Autodesk Inventor part; units mm, degrees
ref_plane "YZ Plane" through (0, 0, 0) normal (1, 0, 0) x (0, 1, 0)
ref_plane "XZ Plane" through (0, 0, 0) normal (0, 1, 0) x (-1, 0, 0)
ref_plane "XY Plane" through (0, 0, 0) normal (0, 0, 1) x (1, 0, 0)
sketch "Sketch1" plane through (0, 0, 0) normal (0, 0, 1) x (1, 0, 0)
  line L0 (0, 0) -> (128, 0)
  line L1 (128, 0) -> (128, 22.5)
  line L2 (0, 23.5) -> (0, 0)
  line L3 (68, 23.5) -> (68, 22.5)
  line L4 (68, 22.5) -> (128, 22.5)
  line L5 (33, 23.5) -> (33, 14.5)
  line L6 (33, 14.5) -> (44, 14.5)
  line L7 (44, 14.5) -> (44, 23.5)
  line L8 (68, 23.5) -> (44, 23.5)
  line L9 (33, 23.5) -> (0, 23.5)
  line L10 (72, 14.5) -> (72, 8)
  line L11 (72, 8) -> (76, 4)
  line L12 (76, 4) -> (118, 4)
  line L13 (118, 4) -> (122, 8)
  line L14 (122, 8) -> (122, 14.5)
  line L15 (122, 14.5) -> (118, 18.5)
  line L16 (118, 18.5) -> (76, 18.5)
  line L17 (76, 18.5) -> (72, 14.5)
  line L18 (68, 22.5) -> (68, 0) construction
  circle A0 centre (5.5, 19) radius 2.25
  circle A1 centre (25.5, 19) radius 2.25
  circle A2 centre (15.5, 19.599) radius 2.75
  circle A3 centre (38.5, 19.599) radius 7.5 construction
  circle A4 centre (38.5, 19.599) radius 4 construction
  point P0 (33, 19)
  dimension "d0" = 128
  dimension "d1" = 23.5
  dimension "d2" = 22.5
  dimension "d3" = 60
  dimension "d4" = 11
  dimension "d5" = 9
  dimension "d6" = 33
  dimension "d7" = 45
  dimension "d8" = 4
  dimension "d9" = 4
  dimension "d10" = 6
  dimension "d11" = 4
  dimension "d12" = 4
  dimension "d13" = 4.5
  dimension "d14" = 4.5
  dimension "d15" = 5.5
  dimension "d16" = 20
  dimension "d17" = 5.5
  dimension "d18" = 8
  dimension "d19" = 15
  dimension "d20" = 10
extrude "Extrusion1" add sketch "Sketch1" along normal blind 6.5
sketch "Sketch2" plane through (0, 0, 6.5) normal (0, 0, 1) x (1, 0, 0)
  line L0 (0, 0) -> (128, 0)
  line L1 (128, 0) -> (128, 22.5)
  line L2 (128, 22.5) -> (68, 22.5)
  line L3 (33, 23.5) -> (0, 23.5)
  line L4 (0, 23.5) -> (0, 0)
  line L5 (25, 23.5) -> (33, 23.5)
  line L6 (33, 23.5) -> (33, 29.5)
  line L7 (31, 31.5) -> (27, 31.5)
  line L8 (25, 29.5) -> (25, 23.5)
  line L9 (94, 22.5) -> (102, 22.5)
  line L10 (102, 22.5) -> (102, 27)
  line L11 (100, 29) -> (96, 29)
  line L12 (94, 27) -> (94, 22.5)
  line L13 (15, 0) -> (23, 0)
  line L14 (23, 0) -> (23, -19)
  line L15 (21, -21) -> (17, -21)
  line L16 (15, -19) -> (15, 0)
  line L17 (44, 0) -> (52, 0)
  line L18 (52, 0) -> (52, -19)
  line L19 (50, -21) -> (46, -21)
  line L20 (44, -19) -> (44, 0)
  line L21 (94, 0) -> (102, 0)
  line L22 (102, 0) -> (102, -4.5)
  line L23 (100, -6.5) -> (96, -6.5)
  line L24 (94, -4.5) -> (94, 0)
  arc A0 (27, 31.5) -> (25, 29.5) centre (27, 29.5) ccw
  arc A1 (33, 29.5) -> (31, 31.5) centre (31, 29.5) ccw
  arc A2 (96, 29) -> (94, 27) centre (96, 27) ccw
  arc A3 (102, 27) -> (100, 29) centre (100, 27) ccw
  arc A4 (15, -19) -> (17, -21) centre (17, -19) ccw
  arc A5 (21, -21) -> (23, -19) centre (21, -19) ccw
  arc A6 (44, -19) -> (46, -21) centre (46, -19) ccw
  arc A7 (50, -21) -> (52, -19) centre (50, -19) ccw
  arc A8 (94, -4.5) -> (96, -6.5) centre (96, -4.5) ccw
  arc A9 (100, -6.5) -> (102, -4.5) centre (100, -4.5) ccw
  line L25 (33, 14.5) -> (33, 23.5)
  dimension "d23" = 2
  dimension "d24" = 8
  dimension "d25" = 8
  dimension "d26" = 8
  dimension "d27" = 8
  dimension "d28" = 8
  dimension "d29" = 21
  dimension "d30" = 8
  dimension "d31" = 6.5
  dimension "d33" = 26
  dimension "d34" = 15
  dimension "d35" = 21
  dimension "d38" = 6.5
extrude "Extrusion2" add sketch "Sketch2" against normal blind 6.5
properties part number "x_iddler_upper_nut_stop" material "Plywood, Finish"
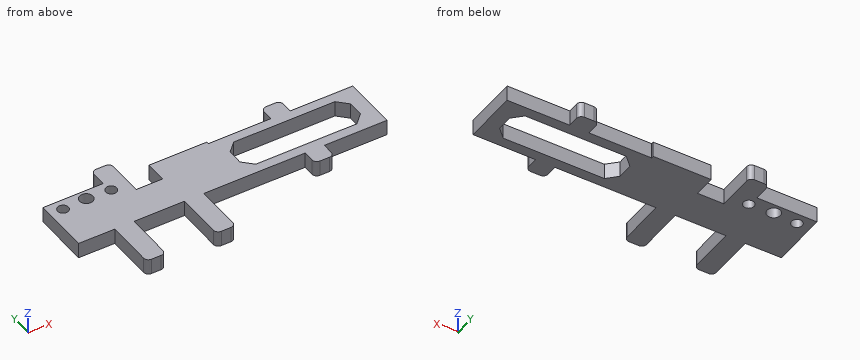
Part model, mm, in its own coordinate system. Coordinates: 2 decimals unless noted, no trailing zeros. Loops run counter-clockwise (first coordinate to the right, second up) from the corner with the lowest first, then second, coordinate; pieces in that order, holes last. Notation, with made-up numbers: (27, 0.5) -> (86, 0.5) arc R16 cw to (86, 7.5) -> close; hole circle Ø5 at (49.5, 28.25). An arc over 180 degrees is marked (long way). Use a Markdown table: item, result. Add a question column.
Item 1: Probe probe 1 along X at (y, z) = (-9, 2.5); probe 2 along X at (y, z) = (16, 3.5); probe 3 along X at (y, z) = (24.5, 1.5). List the from-to ranges inside material, lowest first.
Item 2: Flat gauge pins, fed straight in: P1, Ø3, axis at y = -13.5, z = 2, coming from the +X side; P2, Ø1.8, axis at y = 27.5, z = 5, coming from the -X side; P3, Ø2, axis at y = -5, z = 2.5, coming from the +X side; P4, Ø3.5, axis at x = 25.5, y = 19, coming from the -Z side. Where does each tip first touch, or does it go through?
Item 3: Band-saw the part on C-C on y = -3. Write the cut outline in (x, z), plus the area to 3 significant figures.
Item 4: Band-saw the part on B-B on y = 12. Write the cut outline in (x, z), plus the area to 3 significant figures.
Item 5: Band-saw the part on D-D on x = 48.5. Write the cut outline in (y, z), plus the area to 3 significant figures.
Item 6: Band-saw the part on A-A on x = 5.5. Write the cut outline in (y, z), plus the area to 4 significant figures.
Geometry says:
| question | item | result |
|---|---|---|
| 1 | probe 1 | 15 to 23, 44 to 52 |
| 1 | probe 2 | 0 to 33, 44 to 73.5, 120.5 to 128 |
| 1 | probe 3 | 25 to 33, 94 to 102 |
| 2 | P1 | x = 52 |
| 2 | P2 | x = 25 |
| 2 | P3 | x = 102 |
| 2 | P4 | through |
| 3 | outline | (15, 0) -> (23, 0) -> (23, 6.5) -> (15, 6.5) -> close; (44, 0) -> (52, 0) -> (52, 6.5) -> (44, 6.5) -> close; (94, 0) -> (102, 0) -> (102, 6.5) -> (94, 6.5) -> close |
| 3 | area | 156 mm² |
| 4 | outline | (0, 0) -> (72, 0) -> (72, 6.5) -> (0, 6.5) -> close; (122, 0) -> (128, 0) -> (128, 6.5) -> (122, 6.5) -> close |
| 4 | area | 507 mm² |
| 5 | outline | (-21, 0) -> (23.5, 0) -> (23.5, 6.5) -> (-21, 6.5) -> close |
| 5 | area | 289 mm² |
| 6 | outline | (0, 0) -> (16.75, 0) -> (16.75, 6.5) -> (0, 6.5) -> close; (21.25, 0) -> (23.5, 0) -> (23.5, 6.5) -> (21.25, 6.5) -> close |
| 6 | area | 123.5 mm² |
